Read the model definition and answer for the solid it produces. Units are mm, in the model's axes. Face numbers are marked on the shaded views. A direction names the side the tool comes from. Coordinates: 2 decimals unless noted, no trailing zeros. Write each loop counter-clockwise with the first axis right and the second up, starting at its lowest first coordinate (ties: lowest second). Pieces come first, ordered by that corner, then holes.
1) Find the intervals of material crossed by line 1 (X direction, y = -18, z = -15.5); line 2 (X direction, y = 7.5, z = -8.5); line 3 (Y direction, x = 1, z = -22.5), in increasing order.
2) The part is cut by section B-B (y = 0). Determine the outline of the cut face in (x, z), then the cut area to 3 significant figures.
3) The part is cut by section C-C (x = 1.5). Determine the outline of the cut face in (y, z).
4) Which of the six approach directions +Z, -Z, +X, -X, +Y, -Y give full straight-line access (tool end or side, diameter ignored) to the marked faces 1 and 2?
5) The part is cut by section A-A (z = 0). Determine the outline of the cut face in (x, y).
6) The part is cut by section D-D (x = -22). Determine the outline of the cut face in (y, z), then the cut area to 3 significant figures.
7) Each of these flat-tipped pins is pushed along its axis until it touches: pin 1 Ø4 at (y, z) = (16, -4) entering from -X; pin 2 Ø2 at (x, y) = (-3.5, -4) entering from -Z; pin 3 Ø12 at (x, z) = (-0.5, -22.5) entering from +Y. Where does it stop, or does it pass through?
from build123d import *

# Parameters (mm, degrees)
SKETCH_1_R          = 35
SKETCH_1_R_2        = 2
EXTRUDE_1_DEPTH     = 4
SKETCH_2_R          = 12
EXTRUDE_2_DEPTH     = 3
SKETCH_3_R          = 2.5
EXTRUDE_3_DEPTH     = 2
SKETCH_4_R          = 25
EXTRUDE_4_DEPTH     = 25
EXTRUDE_START       = 11
SKETCH_5_R          = 2.5
EXTRUDE_5_DEPTH     = 11
CUT_EXTRUDE_1_DEPTH = 11


with BuildPart() as part:
    # 草图1 → 凸台-拉伸1 (new body)
    with BuildSketch(Plane(origin=(0, 0, 0), x_dir=(0, 0, -1), z_dir=(1, 0, 0))):
        Circle(SKETCH_1_R)
        with Locations((21.213203436, 21.213203436)):
            Circle(SKETCH_1_R_2, mode=Mode.SUBTRACT)
        with Locations((-21.213203436, 21.213203436)):
            Circle(SKETCH_1_R_2, mode=Mode.SUBTRACT)
        with Locations((-21.213203436, -21.213203436)):
            Circle(SKETCH_1_R_2, mode=Mode.SUBTRACT)
        with Locations((21.213203436, -21.213203436)):
            Circle(SKETCH_1_R_2, mode=Mode.SUBTRACT)
    extrude(amount=EXTRUDE_1_DEPTH)

    # 草图2 → 凸台-拉伸2 (add)
    with BuildSketch(Plane(origin=(4, 0, 0), x_dir=(0, 0, -1), z_dir=(1, 0, 0))):
        Circle(SKETCH_2_R)
    extrude(amount=EXTRUDE_2_DEPTH)

    # 草图3 → 凸台-拉伸3 (add)
    with BuildSketch(Plane(origin=(7, 0, 0), x_dir=(0, 0, -1), z_dir=(1, 0, 0))):
        Circle(SKETCH_3_R)
    extrude(amount=EXTRUDE_3_DEPTH)

    # 草图4 → 凸台-拉伸4 (add)
    with BuildSketch(Plane.ZY):
        Circle(SKETCH_4_R)
    extrude(amount=EXTRUDE_4_DEPTH)

    # 草图5 → 凸台-拉伸5 (add)
    with BuildSketch(Plane.ZY.offset(25).offset(EXTRUDE_START)):
        with Locations(Location((0, 0, 0), (0, 0, 180))):
            Circle(SKETCH_5_R)
    extrude(amount=-EXTRUDE_5_DEPTH)

    # 草图6 → 切除-拉伸1 (cut)
    with BuildSketch(Plane.ZY.offset(36)):
        Polygon((1.5, -2), (-1.5, -2), (-1.5, -3.83926129), (2.04191787, -3.83926129), align=None)
    extrude(amount=-CUT_EXTRUDE_1_DEPTH, mode=Mode.SUBTRACT)


solid = part.part
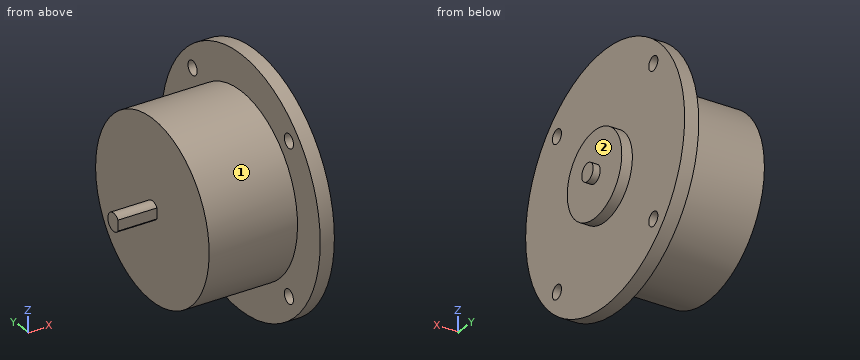
Reported:
1. line 1: x = -25 to 4
1. line 2: x = -25 to 7
1. line 3: y = -26.81 to -22.74, -19.68 to 19.68, 22.74 to 26.81
2. outline: (-36, -2.5) - (-25, -2.5) - (-25, -25) - (0, -25) - (0, -35) - (4, -35) - (4, -12) - (7, -12) - (7, -2.5) - (9, -2.5) - (9, 2.5) - (7, 2.5) - (7, 12) - (4, 12) - (4, 35) - (0, 35) - (0, 25) - (-25, 25) - (-25, 2.5) - (-36, 2.5) - close
2. area: 1,670 mm2
3. outline: circle Ø70 at (0, 0); hole circle Ø4 at (-21.21, -21.21); hole circle Ø4 at (-21.21, 21.21); hole circle Ø4 at (21.21, -21.21); hole circle Ø4 at (21.21, 21.21)
4. face 1: -X
4. face 2: +X
5. outline: (-36, -2) - (-25, -2) - (-25, -25) - (0, -25) - (0, -35) - (4, -35) - (4, -12) - (7, -12) - (7, -2.5) - (9, -2.5) - (9, 2.5) - (7, 2.5) - (7, 12) - (4, 12) - (4, 35) - (0, 35) - (0, 25) - (-25, 25) - (-25, 2.5) - (-36, 2.5) - close
6. outline: circle Ø50 at (0, 0)
6. area: 1,960 mm2
7. pin 1: stops at x = -25
7. pin 2: stops at z = -24.82
7. pin 3: stops at y = 30.86
